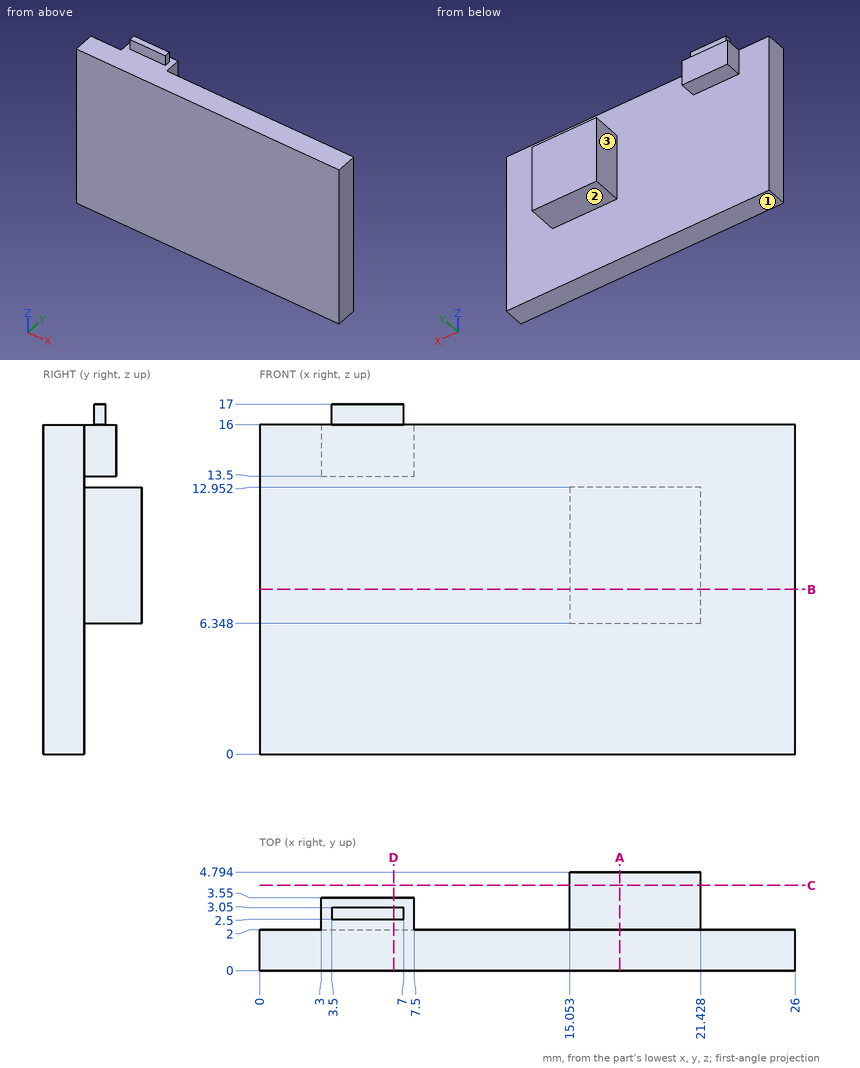
The drawing under review shows one solid part. Ordinate dimensions are in mm from its lowest x, y, z. A direction names the side the tool comes from. Give positions to 0.01 mm unless a question says otherwise; leave off trailing zeros. Write each loop counter-clockwise with the first axis right and the second up, starting at its lowest first coordinate (ties: lowest second). Pieces come first, ordered by that corner, then holes.
1. Add section A-A, the plane x = 17.5. Write out the cut boundary in (y, z).
2. Tool access review of the marked faces 1, 2 and 3: name each direction out of +Z, -Z, +X, -X, +Y, -Y from which nothing blocks a thin tool from reaching the whole face with its end or side.
3. Add section C-C, the plane y = 4.15. Write out the cut boundary in (x, z).
4. For P1, Ø3, axis at x = 5, z = 15, coming from the +Y side; P2, Ø1.2, axis at y = 3, z = 14.5, coming from the -X side; P3, Ø0.8, axis at x = 6, y = 3, coming from the -Z side, all flat-tipped, find the tip position at first contact; note any pin that passes through.
5. Add section D-D, the plane x = 6.5. Write out the cut boundary in (y, z).
6. Add section B-B, the plane z = 8. Write out the cut boundary in (x, y).
7. Wall thickness on L1, parallel to Y at x = 21.75, z = 10.5; L2, parallel to X at y = 3.8, z = 7; L3, parallel to Z at x = 14.75, y = 0.3: over which ranges is each line inside the solid? List them lowest first.
Worked answers:
1. outline: (0, 0) - (2, 0) - (2, 6.35) - (4.79, 6.35) - (4.79, 12.95) - (2, 12.95) - (2, 16) - (0, 16) - close
2. face 1: -Z, +X, -X, +Y, -Y
2. face 2: -Z, +X, -X, +Y
2. face 3: +Z, -Z, -X, +Y
3. outline: (15.05, 6.35) - (21.43, 6.35) - (21.43, 12.95) - (15.05, 12.95) - close
4. P1: stops at y = 3.55
4. P2: stops at x = 3
4. P3: stops at z = 13.5
5. outline: (0, 0) - (2, 0) - (2, 13.5) - (3.55, 13.5) - (3.55, 16) - (3.05, 16) - (3.05, 17) - (2.5, 17) - (2.5, 16) - (0, 16) - close
6. outline: (0, 0) - (26, 0) - (26, 2) - (21.43, 2) - (21.43, 4.79) - (15.05, 4.79) - (15.05, 2) - (0, 2) - close
7. L1: y = 0 to 2
7. L2: x = 15.05 to 21.43
7. L3: z = 0 to 16
